Input: part model. Units: mm. Frame: model coordinates. Face numbers are marked on the shaded views. Round coordinates to 2 decimals unless told otherwise and drop trailing zeros. Loops run counter-clockwise (first coordinate to the right, second up) from the corner with the lowest first, then second, coordinate; pieces in that order, holes last. Notation, with made-up numbers: M 23.5,30.5 L 47.5,30.5 A27 cw 47.5,48.5 Z; hole C 10,-26.75 d1. An arc over 180 degrees is marked long. Put each result on its own line as item: value. Start each with the question number.
1) Section A-A on x = 54. Output: boundary loops of the cut face in (y, z), plus the area to 3 significant figures.
2) Section C-C on z = 0.45. State how many separate pieces and enclosed holes the cut face has, plus the area to 3 significant figures.
3) Line query: probe 1 along X at (y, z) = (-3.5, 0.35); probe 2 along X at (y, z) = (-40, 0.5); probe 3 along X at (y, z) = (7.5, 0.8). Output: solid intervals per line, ascending.
4) Section B-B on y = 46.5. Output: boundary loops of the cut face in (x, z), plus the area to 3 significant figures.
5) Draft query along Z for the marked faces 1 and 2. Return one class per face: +Z half, -Z half, draft (parallel to the pull), parting line (faces both ways), or undercut.
6) Pin query (flat end, axial travel): pin 1 (0.5 mm diameter, centred on y = -46.5, z = 1, fed in from -X); pin 2 (0.8 mm diameter, centred on x = 1, z = 1, fed in from +Y); pin 3 (0.8 mm diameter, centred on x = 0.5, z = 1, fed in from -Y). Return the tip coordinate at first contact, or that it passes through.
from build123d import *

# Parameters (mm, degrees)
MODEL_R             = 1
MODEL_R_2           = 0.5
MODEL_R_3           = 0.35
MODEL_W             = 9.2
MODEL_H             = 16.2
BOSS_EXTRUDE1_DEPTH = 1.6


with BuildPart() as part:
    # Model → Boss-Extrude1 (new body)
    with BuildSketch(Plane.XY):
        Polygon((-78.78461875, -13.89185), (-69.28203125, -40), (-51.423009375, -61.283559375), (-27.361609375, -75.175409375), (0, -80), (27.361609375, -75.175409375), (51.423009375, -61.283559375), (69.28203125, -40), (78.78461875, -13.89185), (78.78461875, 13.89185), (69.28203125, 40), (51.423009375, 61.283559375), (27.361609375, 75.175409375), (0, 80), (-27.361609375, 75.175409375), (-51.423009375, 61.283559375), (-69.28203125, 40), (-78.78461875, 13.89185), align=None)
        with Locations((34.64, -60)):
            Circle(MODEL_R, mode=Mode.SUBTRACT)
        with Locations((-34.64, 60.01)):
            Circle(MODEL_R, mode=Mode.SUBTRACT)
        with Locations((34.65, 60)):
            Circle(MODEL_R, mode=Mode.SUBTRACT)
        with Locations((-34.64, -60)):
            Circle(MODEL_R, mode=Mode.SUBTRACT)
        with Locations((6.3176, -61.378)):
            Circle(MODEL_R_2, mode=Mode.SUBTRACT)
        with Locations((6.3176, -63.918)):
            Circle(MODEL_R_2, mode=Mode.SUBTRACT)
        with Locations((3.7776, -63.918)):
            Circle(MODEL_R_2, mode=Mode.SUBTRACT)
        with Locations((1.2376, -63.918)):
            Circle(MODEL_R_2, mode=Mode.SUBTRACT)
        with Locations((2.5374, -27.5374)):
            Circle(MODEL_R_2, mode=Mode.SUBTRACT)
        with Locations((-0.0026, -27.5374)):
            Circle(MODEL_R_2, mode=Mode.SUBTRACT)
        with Locations((-2.5426, -27.5374)):
            Circle(MODEL_R_2, mode=Mode.SUBTRACT)
        with Locations((-2.5426, -24.9974)):
            Circle(MODEL_R_2, mode=Mode.SUBTRACT)
        with Locations((2.5374, -24.9974)):
            Circle(MODEL_R_2, mode=Mode.SUBTRACT)
        with Locations((-3.5074, -63.9222)):
            Circle(MODEL_R_2, mode=Mode.SUBTRACT)
        with Locations((-6.0474, -63.9222)):
            Circle(MODEL_R_2, mode=Mode.SUBTRACT)
        with Locations((-8.5874, -63.9222)):
            Circle(MODEL_R_2, mode=Mode.SUBTRACT)
        with Locations((-8.5874, -61.3822)):
            Circle(MODEL_R_2, mode=Mode.SUBTRACT)
        with Locations((-6.0474, -61.3822)):
            Circle(MODEL_R_2, mode=Mode.SUBTRACT)
        with Locations((-3.5074, -61.3822)):
            Circle(MODEL_R_2, mode=Mode.SUBTRACT)
        with Locations((-0.0026, -24.9974)):
            Circle(MODEL_R_2, mode=Mode.SUBTRACT)
        with Locations((1.2376, -61.378)):
            Circle(MODEL_R_2, mode=Mode.SUBTRACT)
        with Locations((3.7776, -61.378)):
            Circle(MODEL_R_2, mode=Mode.SUBTRACT)
        with Locations((-5.35, -43.105)):
            Circle(MODEL_R_3, mode=Mode.SUBTRACT)
        with Locations((-5.35, -44.885)):
            Circle(MODEL_R_3, mode=Mode.SUBTRACT)
        with Locations((-5.35, -46.665)):
            Circle(MODEL_R_3, mode=Mode.SUBTRACT)
        with Locations((-5.35, -48.445)):
            Circle(MODEL_R_3, mode=Mode.SUBTRACT)
        with Locations((-5.35, -50.225)):
            Circle(MODEL_R_3, mode=Mode.SUBTRACT)
        with Locations((-5.35, -52.005)):
            Circle(MODEL_R_3, mode=Mode.SUBTRACT)
        with Locations((-5.35, -53.785)):
            Circle(MODEL_R_3, mode=Mode.SUBTRACT)
        with Locations((5.35, -54.675)):
            Circle(MODEL_R_3, mode=Mode.SUBTRACT)
        with Locations((5.35, -52.895)):
            Circle(MODEL_R_3, mode=Mode.SUBTRACT)
        with Locations((5.35, -51.115)):
            Circle(MODEL_R_3, mode=Mode.SUBTRACT)
        with Locations((5.35, -49.335)):
            Circle(MODEL_R_3, mode=Mode.SUBTRACT)
        with Locations((5.35, -47.555)):
            Circle(MODEL_R_3, mode=Mode.SUBTRACT)
        with Locations((5.35, -45.775)):
            Circle(MODEL_R_3, mode=Mode.SUBTRACT)
        with Locations((5.35, -43.995)):
            Circle(MODEL_R_3, mode=Mode.SUBTRACT)
        with Locations((-5.35, -41.325)):
            Circle(MODEL_R_3, mode=Mode.SUBTRACT)
        with Locations((5.35, -42.215)):
            Circle(MODEL_R_3, mode=Mode.SUBTRACT)
        with Locations((0, -47.9)):
            Rectangle(MODEL_W, MODEL_H, mode=Mode.SUBTRACT)
        Polygon((-72.28461875, -12.74573125), (-63.56603125, -36.699859375), (-47.180440625, -56.22745), (-39.389909375, -60.72531875), (-37.45445, -58.37865), (-35.482740625, -56.865709375), (-33.01871875, -57.1901), (-31.50578125, -59.161809375), (-31.83016875, -61.62583125), (-32.894709375, -64.47531875), (-25.104190625, -68.97318125), (-19.53553125, -69.955090625), (-16, -66.41955), (-16, 3.4641), (-61.494659375, 29.730459375), (-66.4187, 28.86221875), (-72.28461875, 12.74573125), align=None, mode=Mode.SUBTRACT)
        Polygon((16, -66.41955), (19.53553125, -69.955090625), (25.104190625, -68.97318125), (32.894709375, -64.47531875), (31.83016875, -61.62583125), (31.50578125, -59.161809375), (33.01871875, -57.1901), (35.482740625, -56.865709375), (37.45445, -58.37865), (39.389909375, -60.72531875), (47.180440625, -56.22745), (63.56603125, -36.699859375), (72.28461875, -12.74573125), (72.28461875, 12.74573125), (66.4187, 28.86221875), (61.494659375, 29.730459375), (16, 3.4641), align=None, mode=Mode.SUBTRACT)
        Polygon((-57.802509375, 43.568559375), (-56.93426875, 38.64451875), (-5, 8.66025), (5, 8.66025), (56.93426875, 38.64451875), (57.802509375, 43.568559375), (47.180440625, 56.22745), (39.389909375, 60.72531875), (37.45445, 58.37865), (35.482740625, 56.865709375), (33.01871875, 57.1901), (31.50578125, 59.161809375), (31.83016875, 61.62583125), (32.894709375, 64.47531875), (25.104190625, 68.97318125), (0, 73.39973125), (-25.104190625, 68.97318125), (-32.894709375, 64.47531875), (-31.83016875, 61.62583125), (-31.50578125, 59.161809375), (-33.01871875, 57.1901), (-35.482740625, 56.865709375), (-37.45445, 58.37865), (-39.389909375, 60.72531875), (-47.180440625, 56.22745), align=None, mode=Mode.SUBTRACT)
    extrude(amount=BOSS_EXTRUDE1_DEPTH)


solid = part.part
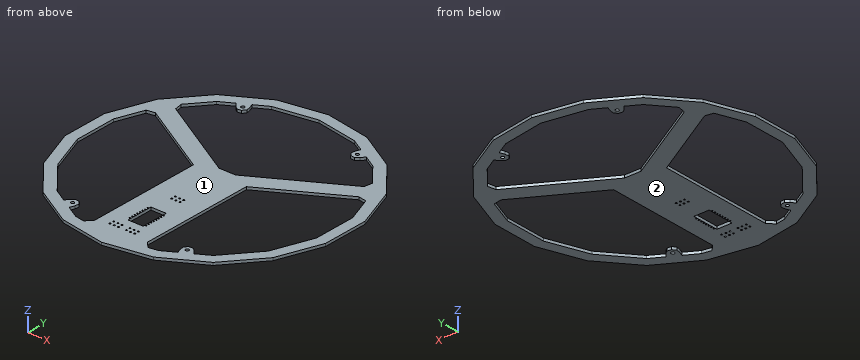
Geometry results:
1. outline: M -58.21,0 L -48.1,0 L -48.1,1.6 L -58.21,1.6 Z; M 25.4,0 L 36.95,0 L 36.95,1.6 L 25.4,1.6 Z; M 48.1,0 L 58.21,0 L 58.21,1.6 L 48.1,1.6 Z
1. area: 50.8 mm²
2. separate pieces: 1
2. enclosed holes: 42
2. area: 6,860 mm²
3. probe 1: x = -78.78 to -72.28, -16 to 16, 72.28 to 78.78
3. probe 2: x = -69.28 to -60.8, -16 to -4.6, 4.6 to 16, 60.8 to 69.28
3. probe 3: x = -78.78 to -72.28, -22.99 to 22.99, 72.28 to 78.78
4. outline: M -63.83,0 L -55.34,0 L -55.34,1.6 L -63.83,1.6 Z; M 55.34,0 L 63.83,0 L 63.83,1.6 L 55.34,1.6 Z
4. area: 27.2 mm²
5. face 1: +Z half
5. face 2: -Z half
6. pin 1: stops at x = -64.04
6. pin 2: stops at y = 79.89
6. pin 3: stops at y = -79.98
